```python
from build123d import *

# Parameters (mm, degrees)
SKETCH2_R           = 2.65
BOSS_EXTRUDE1_DEPTH = 200


with BuildPart() as part:
    # Sketch2 → Boss-Extrude1 (new body)
    with BuildSketch(Plane.XY):
        with BuildLine():
            Line((0, 2), (0, 8.007512652))
            ThreePointArc((0, 8.007512652), (0.146446609, 8.361066043), (0.5, 8.507512652))
            Line((0.5, 8.507512652), (1.5, 8.507512652))
            ThreePointArc((1.5, 8.507512652), (1.853553391, 8.361066043), (2, 8.007512652))
            Line((2, 8.007512652), (2, 5.451323229))
            ThreePointArc((2, 5.451323229), (2.301581692, 4.992378598), (2.842520699, 5.087071159))
            Line((2.842520699, 5.087071159), (6.485041399, 8.512278154))
            Line((6.485041399, 8.512278154), (6.485041399, 11.512278154))
            Line((6.485041399, 11.512278154), (2.842520699, 14.937485148))
            ThreePointArc((2.842520699, 14.937485148), (2.301581692, 15.03217771), (2, 14.573233078))
            Line((2, 14.573233078), (2, 13.307512652))
            ThreePointArc((2, 13.307512652), (1.853553391, 12.953959262), (1.5, 12.807512652))
            Line((1.5, 12.807512652), (0.5, 12.807512652))
            ThreePointArc((0.5, 12.807512652), (0.146446609, 12.953959262), (0, 13.307512652))
            Line((0, 13.307512652), (0, 18))
            ThreePointArc((0, 18), (0.585786438, 19.414213562), (2, 20))
            Line((2, 20), (6.5, 20))
            ThreePointArc((6.5, 20), (6.853553391, 19.853553391), (7, 19.5))
            Line((7, 19.5), (7, 18.017502122))
            ThreePointArc((7, 18.017502122), (6.853553391, 17.663948732), (6.5, 17.517502122))
            Line((6.5, 17.517502122), (5.2, 17.517502122))
            ThreePointArc((5.2, 17.517502122), (4.735174207, 17.201722052), (4.857479301, 16.653250052))
            Line((4.857479301, 16.653250052), (8.5, 13.228043058))
            Line((8.5, 13.228043058), (11.5, 13.228043058))
            Line((11.5, 13.228043058), (15.142520699, 16.653250052))
            ThreePointArc((15.142520699, 16.653250052), (15.264825793, 17.201722052), (14.8, 17.517502122))
            Line((14.8, 17.517502122), (13.5, 17.517502122))
            ThreePointArc((13.5, 17.517502122), (13.146446609, 17.663948732), (13, 18.017502122))
            Line((13, 18.017502122), (13, 19.5))
            ThreePointArc((13, 19.5), (13.146446609, 19.853553391), (13.5, 20))
            Line((13.5, 20), (18, 20))
            ThreePointArc((18, 20), (19.414213562, 19.414213562), (20, 18))
            Line((20, 18), (20, 13.307512652))
            ThreePointArc((20, 13.307512652), (19.853553391, 12.953959262), (19.5, 12.807512652))
            Line((19.5, 12.807512652), (18.5, 12.807512652))
            ThreePointArc((18.5, 12.807512652), (18.146446609, 12.953959262), (18, 13.307512652))
            Line((18, 13.307512652), (18, 14.573233078))
            ThreePointArc((18, 14.573233078), (17.698418308, 15.03217771), (17.157479301, 14.937485148))
            Line((17.157479301, 14.937485148), (13.514958601, 11.512278154))
            Line((13.514958601, 11.512278154), (13.514958601, 8.512278154))
            Line((13.514958601, 8.512278154), (17.157479301, 5.087071159))
            ThreePointArc((17.157479301, 5.087071159), (17.698418308, 4.992378598), (18, 5.451323229))
            Line((18, 5.451323229), (18, 8.007512652))
            ThreePointArc((18, 8.007512652), (18.146446609, 8.361066043), (18.5, 8.507512652))
            Line((18.5, 8.507512652), (19.5, 8.507512652))
            ThreePointArc((19.5, 8.507512652), (19.853553391, 8.361066043), (20, 8.007512652))
            Line((20, 8.007512652), (20, 2))
            ThreePointArc((20, 2), (19.414213562, 0.585786438), (18, 0))
            Line((18, 0), (13.5, 0))
            ThreePointArc((13.5, 0), (13.146446609, 0.146446609), (13, 0.5))
            Line((13, 0.5), (13, 2.007054185))
            ThreePointArc((13, 2.007054185), (13.146446609, 2.360607576), (13.5, 2.507054185))
            Line((13.5, 2.507054185), (14.8, 2.507054185))
            ThreePointArc((14.8, 2.507054185), (15.264825793, 2.822834256), (15.142520699, 3.371306255))
            Line((15.142520699, 3.371306255), (11.5, 6.79651325))
            Line((11.5, 6.79651325), (8.5, 6.79651325))
            Line((8.5, 6.79651325), (4.857479301, 3.371306255))
            ThreePointArc((4.857479301, 3.371306255), (4.735174207, 2.822834256), (5.2, 2.507054185))
            Line((5.2, 2.507054185), (6.5, 2.507054185))
            ThreePointArc((6.5, 2.507054185), (6.853553391, 2.360607576), (7, 2.007054185))
            Line((7, 2.007054185), (7, 0.5))
            ThreePointArc((7, 0.5), (6.853553391, 0.146446609), (6.5, 0))
            Line((6.5, 0), (2, 0))
            ThreePointArc((2, 0), (0.585786438, 0.585786438), (0, 2))
        make_face()
        with Locations((10, 10)):
            Circle(SKETCH2_R, mode=Mode.SUBTRACT)
    extrude(amount=BOSS_EXTRUDE1_DEPTH)


solid = part.part
```
Can you work these out from the model? Positions are in its coordinate system, mm. A direction names the side the tool comes from. Give positions to 0.01 mm unless a question says otherwise; leave off trailing zeros. Use a Markdown table: item, result. Add a question column.
Q1. If we mould it in two halves opening along Y, with no side actions, what happens to faces 1 (the flat face through (4, 0, 99)), 2 (the flat face through (8, 12, 200)), 3 (the flat face through (4.69, 13.2, 98.6))? For each: released by +Y, released by -Y, zero draft, split by the parting line, or undercut.
Q2. I'm going to push flat-ended pins straight in: pin 1 (0.9 mm diameter, centred on x = 9.5, z = 75.5, fed in from -Y); pin 2 (0.5 mm diameter, centred on x = 1, z = 70.5, fed in from -Y); pin 3 (0.5 mm diameter, centred on y = 1.5, z = 84.5, fed in from +X). Where does each tip first touch, or does it pass through?
Q3. Please list where these lines run through material, in increasing order: line 1 along Y through (x, z) = (10, 118); line 2 along X through (y, z) = (1.75, 160); line 3 along X through (y, z) = (6.75, 36).
Q4. On a 3-axis mill with a long thin cutter (end or side, diameter ignored), from which of +Z, -Z, +X, -X, +Y, -Y can I reach the whole of each face in a straight line? I mean faces 4 (the flat face through (16, 0, 99)), 5 (the flat face through (6.653, 14.965, 98.6)). Say none if no direction works.
Answers follow:
| question | item | result |
|---|---|---|
| 1 | face 1 | released by -Y |
| 1 | face 2 | zero draft |
| 1 | face 3 | undercut |
| 2 | pin 1 | stops at y = 6.8 |
| 2 | pin 2 | stops at y = 0.15 |
| 2 | pin 3 | stops at x = 19.98 |
| 3 | line 1 | y = 6.8 to 7.35, 12.65 to 13.23 |
| 3 | line 2 | x = 0.02 to 7, 13 to 19.98 |
| 3 | line 3 | x = 0 to 2, 4.61 to 8.45, 11.55 to 15.39, 18 to 20 |
| 4 | face 4 | +Z, -Z, +X, -X, -Y |
| 4 | face 5 | +Z, -Z |
